Source: CAD feature listing. Evaluate the final solid. Frame: model axes, mm. A direction names the side the tool comes from. Give positions to 0.01 mm unless a question says otherwise; leave off trailing zeros. Order: outer loops, then holes, each group sorted by start corner. A loop starts at its lowest first (then second) coordinate and runs counter-clockwise, first axis right, second up. Notation, with made-up numbers: (7, 88.5) -> (59, 88.5) arc R25 ccw to (59, 121.5) -> close; hole circle Ø10 at (23.25, 2). An arc over 180 degrees is marked (long way). Answer in a Markdown table with one row per item.
```python
from build123d import *

# Parameters (mm, degrees)
F0_W     = 9.62
F0_H     = 28.5
F1_DEPTH = 1.5
F2_W     = 12.62
F2_H     = 31.5
F2_W_2   = 9.62
F2_H_2   = 28.5
F3_DEPTH = 7.3
F4_W     = 12.62
F4_H     = 31.5
F5_DEPTH = 2
F6_W     = 5
F6_H     = 22
F7_DEPTH = 25
F8_R     = 1.6
F9_DEPTH = 25
F10_SIZE = 0.75
F11_SIZE = 0.5


with BuildPart() as f1:
    # F0 (on Top) → F1 (new body)
    with BuildSketch(Plane.XY):
        with BuildLine():
            Line((2.81, 22.25), (-2.81, 22.25))
            ThreePointArc((-2.81, 22.25), (-6.345534, 20.785534), (-7.81, 17.25))
            Line((-7.81, 17.25), (-7.81, -17.25))
            ThreePointArc((-7.81, -17.25), (-6.345534, -20.785534), (-2.81, -22.25))
            Line((-2.81, -22.25), (2.81, -22.25))
            ThreePointArc((2.81, -22.25), (6.345534, -20.785534), (7.81, -17.25))
            Line((7.81, -17.25), (7.81, 17.25))
            ThreePointArc((7.81, 17.25), (6.345534, 20.785534), (2.81, 22.25))
        make_face()
        Rectangle(F0_W, F0_H, mode=Mode.SUBTRACT)
    extrude(amount=F1_DEPTH)

    # F2 (on face) → F3 (join)
    with BuildSketch(Plane.XY.offset(1.5)):
        Rectangle(F2_W, F2_H)
        Rectangle(F2_W_2, F2_H_2, mode=Mode.SUBTRACT)
    extrude(amount=F3_DEPTH)

    # F4 (on face) → F5 (join)
    with BuildSketch(Plane.XY.offset(8.8)):
        Rectangle(F4_W, F4_H)
    extrude(amount=F5_DEPTH)

    # F6 (on face) → F7 (cut)
    with BuildSketch(Plane.XY.offset(10.8)):
        Rectangle(F6_W, F6_H)
    extrude(amount=-F7_DEPTH, mode=Mode.SUBTRACT)

    # F8 (on face) → F9 (cut)
    with BuildSketch(Plane(origin=(0, 0, 0), x_dir=(1, 0, 0), z_dir=(0, 0, -1))):
        with Locations((0, 18.25)):
            Circle(F8_R)
        with Locations((0, -18.25)):
            Circle(F8_R)
    extrude(amount=-F9_DEPTH, mode=Mode.SUBTRACT)

    # F10
    f10_edges = [f1.edges().sort_by_distance(p)[0] for p in [
        (7.81, 0, 0),
    ]]
    chamfer(f10_edges, length=F10_SIZE)

    # F11
    f11_edges = [f1.edges().sort_by_distance(p)[0] for p in [
        (0, -14.25, 0),
        (4.81, 0, 0),
        (-4.81, 0, 0),
        (0, 14.25, 0),
    ]]
    chamfer(f11_edges, length=F11_SIZE)


solid = f1.part
```
(1) Section query B-B (x = 0). Return the cut outline in (y, z).
A:
| item | result |
|---|---|
| outline | (-22.25, 0.75) -> (-21.5, 0) -> (-19.85, 0) -> (-19.85, 1.5) -> (-22.25, 1.5) -> close; (-16.65, 0) -> (-14.75, 0) -> (-14.25, 0.5) -> (-14.25, 8.8) -> (-11, 8.8) -> (-11, 10.8) -> (-15.75, 10.8) -> (-15.75, 1.5) -> (-16.65, 1.5) -> close; (11, 8.8) -> (14.25, 8.8) -> (14.25, 0.5) -> (14.75, 0) -> (16.65, 0) -> (16.65, 1.5) -> (15.75, 1.5) -> (15.75, 10.8) -> (11, 10.8) -> close; (19.85, 0) -> (21.5, 0) -> (22.25, 0.75) -> (22.25, 1.5) -> (19.85, 1.5) -> close |
(2) Section query C-C (y = -7.5). Return the cut outline in (x, z).
A:
| item | result |
|---|---|
| outline | (-7.81, 0.75) -> (-7.06, 0) -> (-5.31, 0) -> (-4.81, 0.5) -> (-4.81, 8.8) -> (-2.5, 8.8) -> (-2.5, 10.8) -> (-6.31, 10.8) -> (-6.31, 1.5) -> (-7.81, 1.5) -> close; (2.5, 8.8) -> (4.81, 8.8) -> (4.81, 0.5) -> (5.31, 0) -> (7.06, 0) -> (7.81, 0.75) -> (7.81, 1.5) -> (6.31, 1.5) -> (6.31, 10.8) -> (2.5, 10.8) -> close |
(3) Section query D-D (y = -12.5). Return the cut outline in (x, z), plus the area to 3 significant figures.
A:
| item | result |
|---|---|
| outline | (-7.81, 0.75) -> (-7.06, 0) -> (-5.31, 0) -> (-4.81, 0.5) -> (-4.81, 8.8) -> (4.81, 8.8) -> (4.81, 0.5) -> (5.31, 0) -> (7.06, 0) -> (7.81, 0.75) -> (7.81, 1.5) -> (6.31, 1.5) -> (6.31, 10.8) -> (-6.31, 10.8) -> (-6.31, 1.5) -> (-7.81, 1.5) -> close |
| area | 55.3 mm^2 |
(4) Ray query, probe 1 along Y at (x, z) = (0, 1.05); probe 2 along Y at (x, z) = (4.75, 6); probe 3 along X at (y, z) = (-10.5, 6.25). Return the intervals inside material, ascending.
A:
| item | result |
|---|---|
| probe 1 | y = -22.25 to -19.85, -16.65 to -14.25, 14.25 to 16.65, 19.85 to 22.25 |
| probe 2 | y = -15.75 to -14.25, 14.25 to 15.75 |
| probe 3 | x = -6.31 to -4.81, 4.81 to 6.31 |
(5) Section query A-A (z = 6.75). Return the cut outline in (x, y).
A:
| item | result |
|---|---|
| outline | (-6.31, -15.75) -> (6.31, -15.75) -> (6.31, 15.75) -> (-6.31, 15.75) -> close; hole (-4.81, -14.25) -> (4.81, -14.25) -> (4.81, 14.25) -> (-4.81, 14.25) -> close |
(6) First-contact query: pin 1 Ø3 at (y, z) = (2.5, 6.5) entering from +X; pin 2 Ø4.5 at (x, z) = (-2.5, 5.5) entering from +Y; pin 3 Ø1 at (y, z) = (-2, 10) entering from -X. Flat tips, straight axial feed; report the tip coordinate or a pass-through.
A:
| item | result |
|---|---|
| pin 1 | stops at x = 6.31 |
| pin 2 | stops at y = 15.75 |
| pin 3 | stops at x = -6.31 |
(7) Pull-direction query (X, two-part tool) for faces 1 (the flat face through (6, 2, 0)), 2 (the cylindrical face through (-0.208, -19.836, 0.74)), 3 (the conical face through (-5.93, -20.31, 0.12)); classes: +X half, -X half, draft (parallel to the pull), parting line (faces both ways), or undercut.
A:
| item | result |
|---|---|
| face 1 | draft |
| face 2 | undercut |
| face 3 | -X half |
(8) Access query for faces 4 (the flat face through (-4.81, 0, 5)), 5 (the flat face through (0, 11, 10)), 6 (the flat face through (6.31, 0, 6)), 7 (the flat face through (-6.31, 0, 6)). Directions: +Z, -Z, +X, -X, +Y, -Y. A direction counts if a zero-diameter tool reaches every point of the face in a straight line with its end or side. Return the directions, or none.
A:
| item | result |
|---|---|
| face 4 | -Z |
| face 5 | +Z, -Z |
| face 6 | +Z, +X, +Y, -Y |
| face 7 | +Z, -X, +Y, -Y |
